Build history of the part. All positions in model axes, mm. A direction names the side the tool comes from. Coordinates: 2 decimals unless noted, no trailing zeros. Loops run counter-clockwise (first coordinate to the right, second up) from the corner with the lowest first, then second, coordinate; pieces in that order, holes last.
(1) Slice it at A-A (z = 100). Give the cut face in (x, y), and give its area (3 significant figures).
(2) Slice it at D-D (x = 81). Give the cut face in (y, z), and give its area (3 significant figures).
(3) Flat gauge pins, fed straight in: P1, Ø5, axis at y = 224.5, z = 163.5, coming from the -X side; P2, Ø1.5, axis at y = 221, z = 104.5, coming from the -X side; P3, Ø8, axis at y = 137, z = 121.5, coming from the -X side. Where does each tip first touch, or does it go through?
(4) Two-plate mould, pull along X, no slides. Class faces 3 (the face through (230.8, 126.8, 98.6)), 4 (the face through (190, 120, 99)), 5 (the face through (269, 50, 101)): pulls with the +X half, pulls with the -X half, needs draft (parallel to the pull), parting line crosses it, or undercut.
(5) Slice it at C-C (x = 275). Give the cut face in (y, z).
(6) Slice it at B-B (y = 150). Give the cut face in (x, z).
(7) Tool access for faces 1 (the face through (19, 50, 101)), 2 (the face through (148, 0, 99)): list every direction of +Z, -Z, +X, -X, +Y, -Y with a clear straight run to the whole face (end or side of a thin tool).
(8) Wall check: L1, parallel to X at y = 39.5, z = 100; L2, parallel to Z at x = 275, y = 35; L3, parallel to Y at x = 258, z = 165. Give the ranges that are in metal, low to high.
from build123d import *

# Parameters (mm, degrees)
SKETCH1_W           = 300
SKETCH1_H           = 250
BOSS_EXTRUDE1_DEPTH = 200
SKETCH2_W           = 50
SKETCH2_H           = 200
CUT_EXTRUDE1_DEPTH  = 200
SKETCH3_W           = 50
SKETCH3_H           = 200
CUT_EXTRUDE2_DEPTH  = 200
CUT_EXTRUDE3_DEPTH  = 200
CUT_EXTRUDE4_DEPTH  = 200
FILLET1_R           = 64.03882
SKETCH6_R           = 50
CUT_EXTRUDE5_DEPTH  = 200
SKETCH8_R           = 5
CUT_EXTRUDE6_DEPTH  = 200
SKETCH9_R           = 5
CUT_EXTRUDE7_DEPTH  = 200


with BuildPart() as part:
    # Sketch1 → Boss-Extrude1 (new body)
    with BuildSketch(Plane.XY):
        with Locations((150, 125)):
            Rectangle(SKETCH1_W, SKETCH1_H)
    extrude(amount=BOSS_EXTRUDE1_DEPTH)

    # Sketch2 → Cut-Extrude1 (cut)
    with BuildSketch(Plane.XY.offset(200)):
        with Locations((25, 150)):
            Rectangle(SKETCH2_W, SKETCH2_H)
    extrude(amount=-CUT_EXTRUDE1_DEPTH, mode=Mode.SUBTRACT)

    # Sketch3 → Cut-Extrude2 (cut)
    with BuildSketch(Plane.XY.offset(200)):
        with Locations((275, 150)):
            Rectangle(SKETCH3_W, SKETCH3_H)
    extrude(amount=-CUT_EXTRUDE2_DEPTH, mode=Mode.SUBTRACT)

    # Sketch4 → Cut-Extrude3 (cut)
    with BuildSketch(Plane(origin=(0, 0, 0), x_dir=(-1, 0, 0), z_dir=(0, 0, -1))):
        Polygon((-50, 250), (-100, 250), (-50, 50), align=None)
    extrude(amount=-CUT_EXTRUDE3_DEPTH, mode=Mode.SUBTRACT)

    # Sketch5 → Cut-Extrude4 (cut)
    with BuildSketch(Plane(origin=(0, 0, 0), x_dir=(-1, 0, 0), z_dir=(0, 0, -1))):
        Polygon((-250, 250), (-200, 250), (-250, 50), align=None)
    extrude(amount=-CUT_EXTRUDE4_DEPTH, mode=Mode.SUBTRACT)

    # Fillet1
    fillet1_edges = [part.edges().sort_by_distance(p)[0] for p in [
        (100, 250, 100),
        (200, 250, 100),
    ]]
    fillet(fillet1_edges, radius=FILLET1_R)

    # Sketch6 → Cut-Extrude5 (cut)
    with BuildSketch(Plane(origin=(0, 0, 0), x_dir=(-1, 0, 0), z_dir=(0, 0, -1))):
        with Locations((-150, 150)):
            Circle(SKETCH6_R)
    extrude(amount=-CUT_EXTRUDE5_DEPTH, mode=Mode.SUBTRACT)

    # Sketch8 → Cut-Extrude6 (cut)
    with BuildSketch(Plane(origin=(0, 50, 0), x_dir=(1, 0, 0), z_dir=(0, 1, 0))):
        with Locations(Location((25, -100, 0), (0, 0, 270))):
            Circle(SKETCH8_R)
    extrude(amount=-CUT_EXTRUDE6_DEPTH, mode=Mode.SUBTRACT)

    # Sketch9 → Cut-Extrude7 (cut)
    with BuildSketch(Plane(origin=(0, 50, 0), x_dir=(1, 0, 0), z_dir=(0, 1, 0))):
        with Locations(Location((275, -100, 0), (0, 0, 270))):
            Circle(SKETCH9_R)
    extrude(amount=-CUT_EXTRUDE7_DEPTH, mode=Mode.SUBTRACT)


solid = part.part
Response values:
1. outline: (0, 0) - (20, 0) - (20, 50) - (0, 50) - close; (30, 0) - (270, 0) - (270, 50) - (250, 50) - (212.13, 201.49) arc R64.04 ccw to (87.87, 201.49) - (50, 50) - (30, 50) - close; (280, 0) - (300, 0) - (300, 50) - (280, 50) - close; hole circle Ø100 at (150, 150)
1. area: 35,200 mm2
2. outline: (0, 0) - (174, 0) - (174, 200) - (0, 200) - close
2. area: 34,800 mm2
3. P1: stops at x = 97.06
3. P2: stops at x = 95.91
3. P3: stops at x = 70.75
4. face 3: pulls with the +X half
4. face 4: undercut
4. face 5: needs draft
5. outline: (0, 0) - (50, 0) - (50, 95) - (0, 95) - close; (0, 105) - (50, 105) - (50, 200) - (0, 200) - close
6. outline: (75, 0) - (100, 0) - (100, 200) - (75, 200) - close; (200, 0) - (225, 0) - (225, 200) - (200, 200) - close
7. face 1: +Z, -Z, -X, +Y
7. face 2: +Z, -Z, +X, -X, -Y
8. L1: x = 0 to 20, 30 to 270, 280 to 300
8. L2: z = 0 to 95, 105 to 200
8. L3: y = 0 to 50
